Build history of the part. All positions in model axes, mm. Face numbers are marked on the shaded views. Give positions to 0.01 mm unless a question says otherwise; leave off trailing zeros. Write each loop counter-clockwise with the first axis right and the second up, starting at its lowest first coordinate (ties: lowest second). Pieces come first, ordered by that corner, then holes.
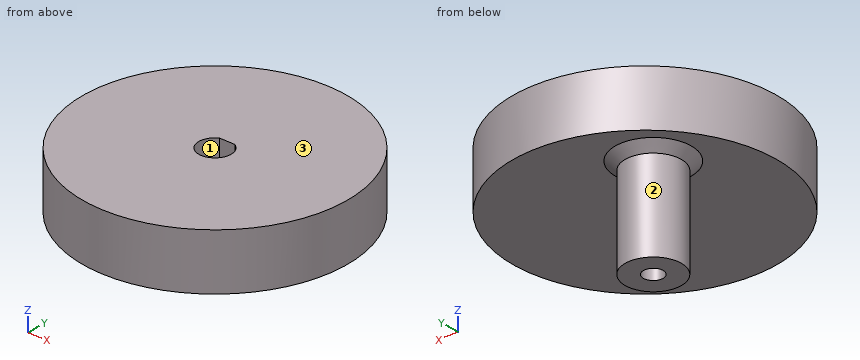
from build123d import *

# Parameters (mm, degrees)
CROQUIS1_R              = 20
SALIENTE_EXTRUIR1_DEPTH = 8.5
CROQUIS2_R              = 4.25
CROQUIS2_R_2            = 1.5
SALIENTE_EXTRUIR2_DEPTH = 15
CHAFL_N1_SIZE           = 1.5
CHAFL_N1_SIZE2          = 1.258649447


with BuildPart() as part:
    # Croquis1 → Saliente-Extruir1 (new body)
    with BuildSketch(Plane.XY):
        Circle(CROQUIS1_R)
        with BuildLine():
            Line((-1.174734012, 2.15), (1.174734012, 2.15))
            ThreePointArc((1.174734012, 2.15), (0, -2.45), (-1.174734012, 2.15))
        make_face(mode=Mode.SUBTRACT)
    extrude(amount=-SALIENTE_EXTRUIR1_DEPTH)

    # Croquis2 → Saliente-Extruir2 (add)
    with BuildSketch(Plane(origin=(0, 0, -8.5), x_dir=(-1, 0, 0), z_dir=(0, 0, -1))):
        with Locations((8.951131501, 8.725092827)):
            Circle(CROQUIS2_R)
        with Locations((8.951131501, 8.725092827)):
            Circle(CROQUIS2_R_2, mode=Mode.SUBTRACT)
    extrude(amount=SALIENTE_EXTRUIR2_DEPTH)

    # Chaflán1
    chafl_n1_edges = [part.edges().sort_by_distance(p)[0] for p in [
        (-4.701131501, 8.725092827, -8.5),
    ]]
    chafl_n1_side = [part.faces().sort_by_distance(p)[0] for p in [
        (-19.434314575, 0, -8.5),
    ]]
    chamfer(chafl_n1_edges, length=CHAFL_N1_SIZE, length2=CHAFL_N1_SIZE2, reference=chafl_n1_side[0])


solid = part.part
1. Saw through at D-D on x = 16. Give the cut face in (y, z), plus the area to 3 significant figures.
2. Drill centre lines: line 1 along Y through (x, z) = (0, -2.25); line 2 along Z through (x, y) = (-6.5, -13); line 3 along X through (y, z) = (8, -16.25). Where is each one in solid material? Low to high.
3. Mould opens along Y. For the marked faces 1, 2 and 3 say: pulls with the +Y half, pulls with the -Y half, needs draft (parallel to the pull), parting line crosses it, or undercut.
4. Saw through at C-C on z = -6. Give the cut face in (x, y), plus the area to 3 significant figures.
5. Saw through at B-B on x = 0. Give the cut face in (y, z).
6. Drop flat-ended pins along their axis: pin 1 (3 mm diameter, centred on x = 2, y = 9, fed in from -Z); pin 2 (2 mm diameter, centred on y = 8, z = -15, fed in from +X); pin 3 (1.5 mm diameter, centred on x = 15, z = -3.5, fed in from -Y). Give the stop position or say it passes through.
7. Saw through at A-A on y = 0. Give the cut face in (x, z), plus the area to 3 significant figures.
Outcome:
1. outline: (-12, -8.5) - (12, -8.5) - (12, 0) - (-12, 0) - close
1. area: 204 mm2
2. line 1: y = -20 to -2.45, 2.15 to 20
2. line 2: z = -8.5 to 0
2. line 3: x = -13.14 to -10.26, -7.64 to -4.76
3. face 1: undercut
3. face 2: parting line crosses it
3. face 3: needs draft
4. outline: circle Ø40 at (0, 0); hole (-1.17, 2.15) arc R2.45 ccw (long way) to (1.17, 2.15) - close
4. area: 1,240 mm2
5. outline: (-20, -8.5) - (-2.45, -8.5) - (-2.45, 0) - (-20, 0) - close; (2.15, -8.5) - (20, -8.5) - (20, 0) - (2.15, 0) - close
6. pin 1: stops at z = -8.5
6. pin 2: stops at x = -4.7
6. pin 3: stops at y = -14.03
7. outline: (-20, -8.5) - (-2.45, -8.5) - (-2.45, 0) - (-20, 0) - close; (2.45, -8.5) - (20, -8.5) - (20, 0) - (2.45, 0) - close
7. area: 298 mm2
